Source: three-view drawing plus pictorial views. Frame: mm from the lowest corner of the part. A direction names the side the tool comes from. Round coordinates to 2 decimals unless told otherwise and drop trailing zeros. Write each loop counter-clockwise with the first axis right and the second up, starting at its lowest first coordinate (ties: lowest second). Pieces come first, ordered by that corner, then holes. Notation, with made-up numbers: M 64,-23.5 L 113,-23.5 A16 ccw 113,4.5 Z; hole C 59,48.25 d5. An arc over 180 degrees is marked long. Answer as CSV lines item,"result". Start each with the question number.
Q1. Section query A-A on y = 6.5. Output: boundary loops of the cut face in (x, z).
Q2. Section query B-B on x = 9. Output: boundary loops of the cut face in (y, z).
Q3. Section query C-C on y = 3. Output: boundary loops of the cut face in (x, z).
Q4. Ray query, probe 1 along Z at (x, y) = (16, 6.5) (1 decimal); probe 2 along X at (y, z) = (8.5, 27.5); probe 3 along Z at (x, y) = (2.75, 9). Return the intervals inside material, ascending.
Q5. Section query D-D on z = 30. Output: boundary loops of the cut face in (x, y), and give its area (3 significant figures).
Q6. Reachability of the marked faces 1, 2, 3, 4 and 5 from +Z, -Z, +X, -X, +Y, -Y: full face, straight path, thin tool, end or side. Return the list, or none.
Q7. First-contact query: pin 1 (9 mm diameter, centred on x = 7.5, z = 23, fed in from +Y); pin 2 (1.5 mm diameter, centred on x = 18.5, z = 5, fed in from -Y); pin 3 (1 mm diameter, centred on y = 3.5, z = 43.5, fed in from -X); pin 4 (2 mm diameter, centred on x = 2.5, y = 5.5, fed in from -Z). Flat tips, straight axial feed; report the tip coordinate or a pass-through.
Q8. Mould query, pull axis Z, two halves, no side actions, for the marked faces 6, 7, 8 and 9. Classes: pulls with the +Z half, pulls with the -Z half, needs draft (parallel to the pull), parting line crosses it, or undercut.
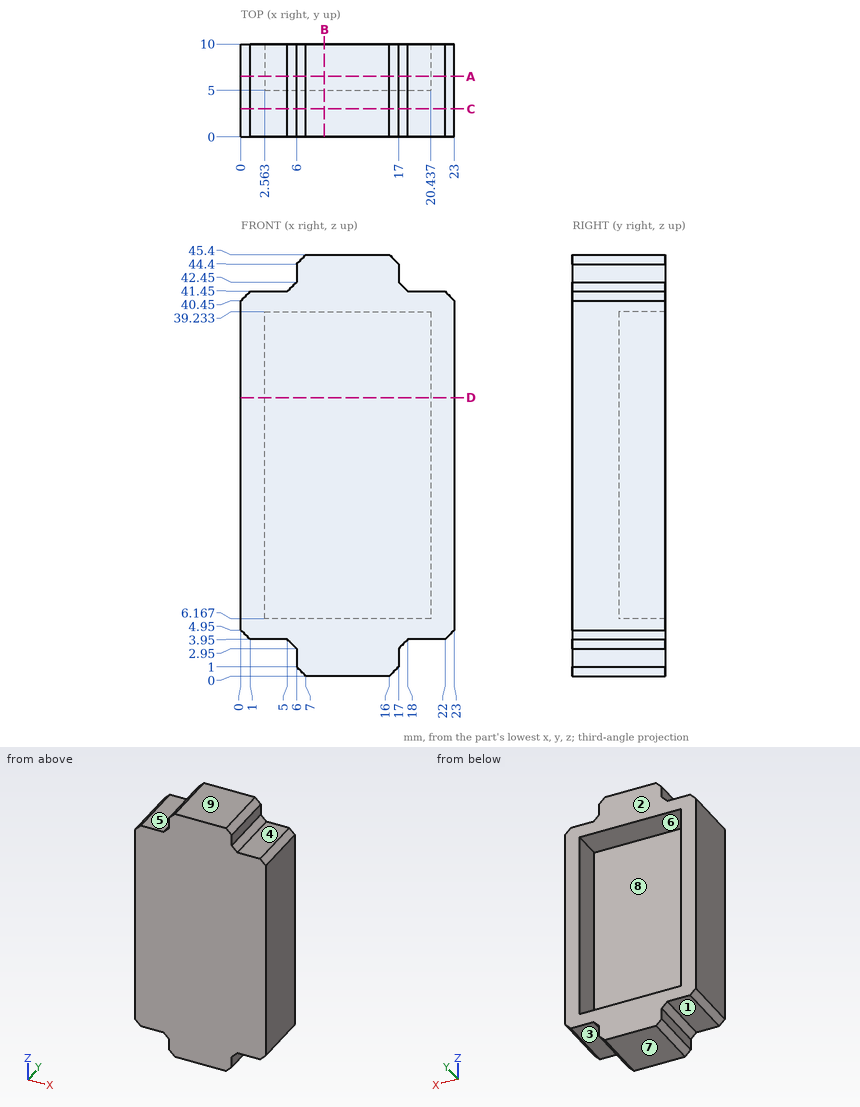
Entries:
1,outline,"M 0,4.95 L 1,3.95 L 5,3.95 L 6,2.95 L 6,1 L 7,0 L 16,0 L 17,1 L 17,2.95 L 18,3.95 L 22,3.95 L 23,4.95 L 23,40.45 L 22,41.45 L 18,41.45 L 17,42.45 L 17,44.4 L 16,45.4 L 7,45.4 L 6,44.4 L 6,42.45 L 5,41.45 L 1,41.45 L 0,40.45 Z; hole M 2.56,6.17 L 20.44,6.17 L 20.44,39.23 L 2.56,39.23 Z"
2,outline,"M 0,0 L 10,0 L 10,6.17 L 5,6.17 L 5,39.23 L 10,39.23 L 10,45.4 L 0,45.4 Z"
3,outline,"M 0,4.95 L 1,3.95 L 5,3.95 L 6,2.95 L 6,1 L 7,0 L 16,0 L 17,1 L 17,2.95 L 18,3.95 L 22,3.95 L 23,4.95 L 23,40.45 L 22,41.45 L 18,41.45 L 17,42.45 L 17,44.4 L 16,45.4 L 7,45.4 L 6,44.4 L 6,42.45 L 5,41.45 L 1,41.45 L 0,40.45 Z"
4,probe 1,"z = 0 to 6.2, 39.2 to 45.4"
4,probe 2,"x = 0 to 2.56, 20.44 to 23"
4,probe 3,"z = 3.95 to 6.17, 39.23 to 41.45"
5,outline,"M 0,0 L 23,0 L 23,10 L 20.44,10 L 20.44,5 L 2.56,5 L 2.56,10 L 0,10 Z"
5,area,"141 mm^2"
6,face 1,"-Z, -X, +Y, -Y"
6,face 2,"+Z, -Z, +X, -X, +Y"
6,face 3,"-Z, +X, +Y, -Y"
6,face 4,"+Z, +X, +Y, -Y"
6,face 5,"+Z, -X, +Y, -Y"
7,pin 1,"stops at y = 5"
7,pin 2,"stops at y = 0"
7,pin 3,"stops at x = 6"
7,pin 4,"stops at z = 3.95"
8,face 6,"undercut"
8,face 7,"pulls with the -Z half"
8,face 8,"undercut"
8,face 9,"pulls with the +Z half"
